Print and shaded views of the part. All mm, measured from the part's lowest x, y and z. A direction names the side the tool comes from. Round coordinates to 2 decimals unless told otherwise and drop trailing zeros. Write each loop counter-clockwise with the first axis right and the second up, starting at its lowest first coordinate (ties: lowest second). Pieces come first, ordered by that corner, then holes.
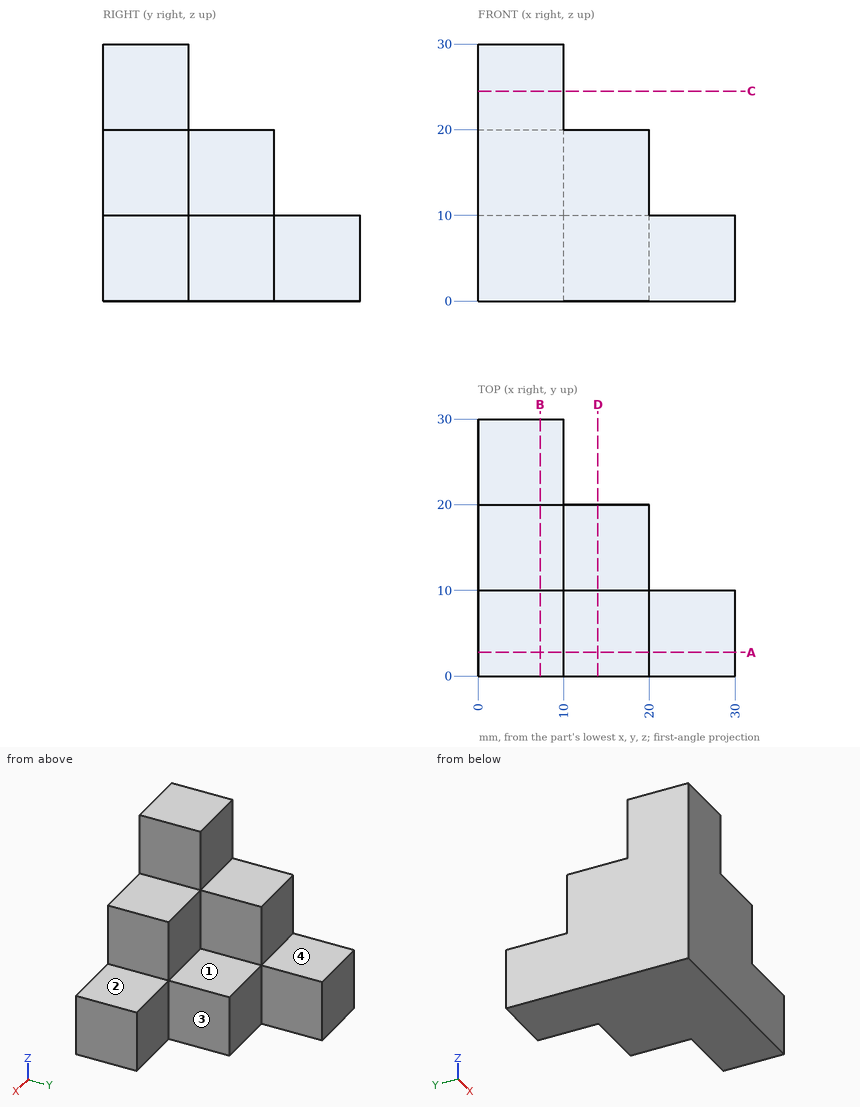
1) Pin check, flat tips, straight feed: pin 1 Ø1.5 at (y, z) = (23.5, 5.5) entering from -X; pin 2 Ø11 at (x, y) = (5.5, 26.5) entering from +Z; pin 3 Ø5 at (x, z) = (13.5, 3) entering from +Y; pin 4 Ø3 at (y, z) = (4.5, 23) entering from +X. Stop position of each tip, or through.
Results:
pin 1: stops at x = 0
pin 2: stops at z = 10
pin 3: stops at y = 20
pin 4: stops at x = 10
2) Which spindle directions (+Z, -Z, +X, -X, +Y, -Y) get a long thin tool onto all of the face, cutting with end or side? Do the marked faces 1, 2, 3 and 4. Say none if no direction does.
Results:
face 1: +Z, +X, +Y
face 2: +Z, +X, +Y, -Y
face 3: +Z, -Z, +X, +Y
face 4: +Z, +X, -X, +Y
3) Slice it at A-A (y = 2.75). Write the cut outline in (x, z), plus the area to 3 significant figures.
Results:
outline: (0, 0) - (30, 0) - (30, 10) - (20, 10) - (20, 20) - (10, 20) - (10, 30) - (0, 30) - close
area: 600 mm2
4) Slice it at D-D (x = 14). Write the cut outline in (y, z), plus the area to 3 significant figures.
Results:
outline: (0, 0) - (20, 0) - (20, 10) - (10, 10) - (10, 20) - (0, 20) - close
area: 300 mm2
5) Slice it at C-C (z = 24.5). Write the cut outline in (x, y), plus the area to 3 significant figures.
Results:
outline: (0, 0) - (10, 0) - (10, 10) - (0, 10) - close
area: 100 mm2
6) Wall check: L1, parallel to X at y = 5.25, z = 26.5. Give the ranges that are in metal, low to high.
Results:
L1: x = 0 to 10
